Autodesk Fusion 360 part; units mm, degrees
sketch "スケッチ1" plane through (0, 0, 0) normal (0, 0, 1) x (1, 0, 0)
  line L0 (0, 0) -> (68.58, 0)
  line L1 (0, 0) -> (68.58, 0)
  line L2 (68.58, 0) -> (68.58, 96.52)
  line L3 (68.58, 96.52) -> (0, 96.52)
  line L4 (0, 96.52) -> (0, 0)
  circle A0 centre (0, 0) radius 1.5
  circle A1 centre (68.58, 0) radius 1.5
  circle A2 centre (0, 96.52) radius 1.5
  circle A3 centre (68.58, 96.52) radius 1.5
  line L5 (-5, -5) -> (73.58, -5)
  line L6 (73.58, -5) -> (73.58, 101.52)
  line L7 (73.58, 101.52) -> (-5, 101.52)
  line L8 (-5, 101.52) -> (-5, -5)
  dimension "d1" = 68.58
  dimension "d2" = 68.58
  dimension "d3" = 96.52
  dimension "d4" = 3
  dimension "d5" = 3
  dimension "d6" = 3
  dimension "d7" = 3
  dimension "d8" = 78.58
  dimension "d9" = 106.52
extrude "押し出し1" add sketch "スケッチ1" along normal blind 2 contours L0 L1 L2 L3 L4 A0 A1 A2 A3 | L5 L6 L7 L8
sketch "スケッチ2" plane through (0, 0, 2) normal (0, 0, 1) x (-1, 0, 0)
  circle A0 centre (0, 0) radius 1.5
  circle A1 centre (-68.58, -96.52) radius 1.5
  circle A2 centre (0, -96.52) radius 1.5
  circle A3 centre (-68.58, 0) radius 1.5
  line L0 (5, -101.52) -> (5, 5)
  line L1 (5, 5) -> (-73.58, 5)
  line L2 (-73.58, 5) -> (-73.58, -101.52)
  line L3 (-73.58, -101.52) -> (5, -101.52)
  line L4 (5, 2.0966) -> (-73.58, 2.0966)
  line L5 (1.9893, 5) -> (1.9893, -101.52)
  line L6 (-70.5693, 5) -> (-70.5693, -101.52)
  line L7 (5, -98.6166) -> (-73.58, -98.6166)
extrude "押し出し2" cut sketch "スケッチ2" against normal blind 2 contours L0 L3 L5 L7 | L0 L4 L5 L7 | L3 L5 L6 L7 | L0 L1 L4 L5 | L2 L3 L6 L7 | L1 L4 L5 L6 | L2 L4 L6 L7 | L1 L2 L4 L6
extrude "押し出し3" cut 1 faces at (45.4465, 32.5919, 2) along direction (0, 0, -1) blind 1
Source: CAD feature listing. Evaluate the final solid. Frame: model axes, mm. Round coordinates to 2 decimals unless told otherwise and drop trailing zeros. Write each loop counter-clockwise with the first axis right and the second up, starting at its lowest first coordinate (ties: lowest second). Pieces come first, ordered by that corner, then holes. Notation, with made-up numbers: M 26.25,72.25 L 45.25,72.25 A17 cw 45.25,79.25 Z; hole C 63.5,40 d2. An arc over 180 degrees is marked long. Answer as a JSON object with one key per item and string values. Group by question number.
(1) Ray query, line 1 (X direction, y = 96.52, z = 0.4); line 2 (Y direction, x = 0, z = 0.7). Return the intervals inside material, ascending. Write a range as [from, to].
(2) Mould query, pull axis X, two halves, no side actions, for faces 1 (the cylindrical face through (67.39, 0.91, 0.49)), 2 (the flat face through (34, 49, 1)), 3 (the cylindrical face through (-1.5, -0.07, 0.49)). Classes: +X half, -X half, draft (parallel to the pull), parting line (faces both ways), or undercut.
(3) First-contact query: pin 1 (6 mm diameter, centred on x = 19.5, y = 12.5, fed in from -Z); pin 2 (1.8 mm diameter, centred on x = 0, y = 0, fed in from -Z). Flat tips, straight axial feed; report the tip coordinate or a pass-through.
(4) Section query B-B on x = 0. Output: boundary loops of the cut face in (y, z), then the cut area to 3 significant figures.
(5) Section query A-A on y = 0. Output: boundary loops of the cut face in (x, z).
Computed values:
{
 "1": {"line 1": "[-1.99, -1.5], [1.5, 67.08], [70.08, 70.57]", "line 2": "[-2.1, -1.5], [1.5, 95.02], [98.02, 98.62]"},
 "2": {"face 1": "undercut", "face 2": "draft", "face 3": "undercut"},
 "3": {"pin 1": "z = 0", "pin 2": "through"},
 "4": {"outline": "M -2.1,0 L -1.5,0 L -1.5,1 L -2.1,1 Z; M 1.5,0 L 95.02,0 L 95.02,1 L 1.5,1 Z; M 98.02,0 L 98.62,0 L 98.62,1 L 98.02,1 Z", "area": "94.7 mm^2"},
 "5": {"outline": "M -1.99,0 L -1.5,0 L -1.5,1 L -1.99,1 Z; M 1.5,0 L 67.08,0 L 67.08,1 L 1.5,1 Z; M 70.08,0 L 70.57,0 L 70.57,1 L 70.08,1 Z"}
}
